Job drawing, mm, ordinate dimensions from the low corner. One solid piece. Round coordinates to 2 decimals unless told otherwise and drop trailing zeros. Order: outer loops, then holes, each group sorted by start corner. A loop starts at its lowest first (then second) coordinate and runs counter-clockwise, first axis right, second up. Notation, with made-up numbers: (66.25, 67) - (88.25, 67) arc R24 ccw to (88.25, 91) - close; hole circle Ø2 at (-36.75, -4). An arc over 180 degrees is marked (long way). Write each question's results on one line, items separated by ' | '. Start each with the question number.
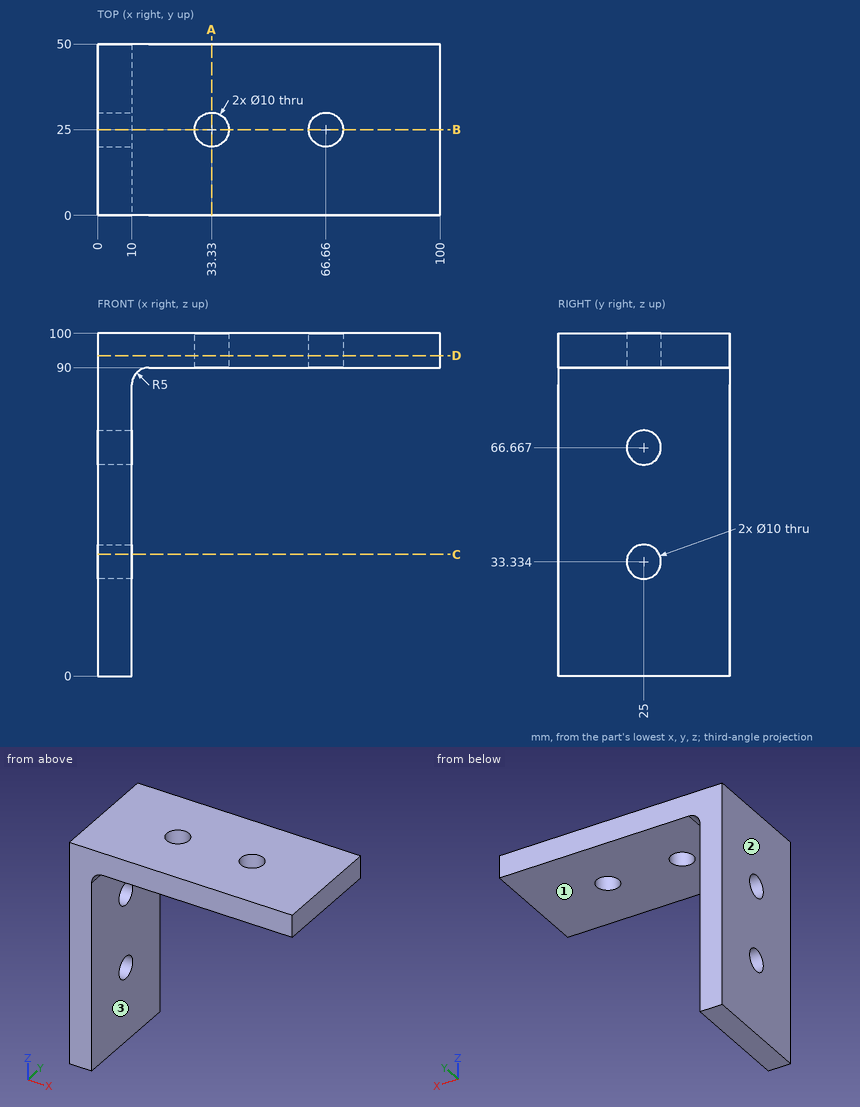
1. Cut at D-D (z = 93.5). List the corners of the cut face in (x, y), plus the area to 3 significant figures.
2. Cut at B-B (y = 25). List the corners of the cut face in (x, z), plus the area to 3 significant figures.
3. Flat gauge pins, fed straight in: pin 1 Ø15 at (y, z) = (14.5, 25) entering from +X; pin 2 Ø1.5 at (x, y) = (17.5, 31) entering from -Z. Where does each tip first touch, or does it go through?
4. Cut at C-C (z = 35.5). List the corners of the cut face in (x, y).
5. Cut at A-A (x = 33.33). List the corners of the cut face in (y, z).
6. Mould opens along X. For the marked faces 1, 2 and 3 say: pulls with the +X half, pulls with the -X half, needs draft (parallel to the pull), parting line crosses it, or undercut.
7. Wall check: line 1 (Y direction, x = 66.66, z = 98); line 2 (X direction, y = 26, z = 17); line 3 (Z direction, x = 21, y = 10). Give the ranges that are in metal, low to high. Write a range as from..to.
A:
1) outline: (0, 0) - (100, 0) - (100, 50) - (0, 50) - close; hole circle Ø10 at (33.33, 25); hole circle Ø10 at (66.66, 25) | area: 4,840 mm^2
2) outline: (0, 0) - (10, 0) - (10, 28.33) - (0, 28.33) - close; (0, 38.33) - (10, 38.33) - (10, 61.67) - (0, 61.67) - close; (0, 71.67) - (10, 71.67) - (10, 85) arc R5 cw to (15, 90) - (28.33, 90) - (28.33, 100) - (0, 100) - close; (38.33, 90) - (61.66, 90) - (61.66, 100) - (38.33, 100) - close; (71.66, 90) - (100, 90) - (100, 100) - (71.66, 100) - close | area: 1,510 mm^2
3) pin 1: stops at x = 10 | pin 2: stops at z = 90
4) outline: (0, 0) - (10, 0) - (10, 20.49) - (0, 20.49) - close; (0, 29.51) - (10, 29.51) - (10, 50) - (0, 50) - close
5) outline: (0, 90) - (20, 90) - (20, 100) - (0, 100) - close; (30, 90) - (50, 90) - (50, 100) - (30, 100) - close
6) face 1: needs draft | face 2: pulls with the -X half | face 3: pulls with the +X half
7) line 1: y = 0..20, 30..50 | line 2: x = 0..10 | line 3: z = 90..100
